```python
from build123d import *

# Parameters (mm, degrees)
SKETCH1_W               = 19.304
SKETCH1_H               = 19.304
BOSS_EXTRUDE1_DEPTH     = 203.2
CUT_EXTRUDE1_DEPTH      = 207.350575478
CUT_EXTRUDE1_DEPTH_BACK = 207.350575478


with BuildPart() as part:
    # Sketch1 → Boss-Extrude1 (new body)
    with BuildSketch(Plane(origin=(0, 0, 0), x_dir=(0, 0, -1), z_dir=(1, 0, 0))):
        with BuildLine():
            Line((0, 2.54), (0, 22.86))
            ThreePointArc((0, 22.86), (-0.743948776, 24.656051224), (-2.54, 25.4))
            Line((-2.54, 25.4), (-22.86, 25.4))
            ThreePointArc((-22.86, 25.4), (-24.656051224, 24.656051224), (-25.4, 22.86))
            Line((-25.4, 22.86), (-25.4, 2.54))
            ThreePointArc((-25.4, 2.54), (-24.656051224, 0.743948776), (-22.86, 0))
            Line((-22.86, 0), (-2.54, 0))
            ThreePointArc((-2.54, 0), (-0.743948776, 0.743948776), (0, 2.54))
        make_face()
        with Locations((-12.7, 12.7)):
            Rectangle(SKETCH1_W, SKETCH1_H, mode=Mode.SUBTRACT)
    extrude(amount=BOSS_EXTRUDE1_DEPTH)

    # Sketch2 → Cut-Extrude1 (cut, two sides: drawn at the far end of the back side and taken through both)
    with BuildSketch(Plane(origin=(0, 25.4, 0), x_dir=(1, 0, 0), z_dir=(0, 1, 0)).offset(-CUT_EXTRUDE1_DEPTH_BACK)):
        with BuildLine():
            Line((203.2, -11.1125), (174.199630657, -11.1125))
            ThreePointArc((174.199630657, -11.1125), (168.275, -12.7), (174.199630657, -14.2875))
            Line((174.199630657, -14.2875), (203.2, -14.2875))
            Line((203.2, -14.2875), (203.2, -11.1125))
        make_face()
    extrude(amount=CUT_EXTRUDE1_DEPTH + CUT_EXTRUDE1_DEPTH_BACK, mode=Mode.SUBTRACT)


solid = part.part
```
Work out the finished part from the listing and answer in its coordinate system (mm). A direction names the side the tool comes from. Give positions to 0.01 mm unless a question says otherwise; leave off trailing zeros. Loops run counter-clockwise (first coordinate to the right, second up) from the corner with the lowest first, then second, coordinate; pieces in that order, holes last. Notation, with made-up numbers: (37, 31.5) -> (72, 31.5) arc R7 ccw to (72, 37.5) -> close; hole circle Ø9 at (15, 76.25). An arc over 180 degrees is marked (long way). Write item = value, one per line. Start each with the question number.
(1) Find the intervals of material crossed by probe 1 along Z at (x, y) = (114.5, 4.5); probe 2 along X at (y, z) = (2.15, 12.7) (3 decimals), in increasing order. Write a range as from..to.
(2) The mould has two halves that part along X. Classify faces 1 (the cylindrical face through (168.277, 1.503, 12.584)), 2 (the flat face through (100, 13, 25.4)), 3 (the flat face through (203.2, 13, 24)): +X half, -X half, draft (parallel to the pull), parting line (faces both ways), or undercut.
(3) Which of the six approach directions +Z, -Z, +X, -X, +Y, -Y give full straight-line access (tool end or side, diameter ignored) to faces 4 (the flat face through (100, 13, 0)), 5 (the flat face through (100, 3.048, 13))?
(4) Find section D-D on x = 25. Give the vertices of the cut face in (y, z), and give its area (3 significant figures).
(5) Find section A-A on x = 171.45. Give the vertices of the cut face in (y, z) (3 decimals).
(6) Given pin 1 Ø2.5 at (x, y) = (185.5, 2) entering from +Z; pin 2 Ø1 at (y, z) = (16.5, 21) entering from +X; pin 3 Ø0.9 at (x, y) = (193, 1.5) entering from -Z, each flat-ended and moving along its own axis, determine where each tip first touches the part or whether it passes through.
(7) Find section B-B on z = 18.5. Give the vertices of the cut face in (x, y), and give its area (3 significant figures).
From the geometry:
q1.probe_1 = 0..3.05, 22.35..25.4
q1.probe_2 = 0..168.275
q2.face_1 = undercut
q2.face_2 = draft
q2.face_3 = +X half
q3.face_4 = -Z, +X, -X, +Y, -Y
q3.face_5 = +X, -X
q4.outline = (0, 2.54) arc R2.54 ccw to (2.54, 0) -> (22.86, 0) arc R2.54 ccw to (25.4, 2.54) -> (25.4, 22.86) arc R2.54 ccw to (22.86, 25.4) -> (2.54, 25.4) arc R2.54 ccw to (0, 22.86) -> close; hole (3.05, 3.05) -> (22.35, 3.05) -> (22.35, 22.35) -> (3.05, 22.35) -> close
q4.area = 267 mm^2
q5.outline = (0, 2.54) arc R2.54 ccw to (2.54, 0) -> (22.86, 0) arc R2.54 ccw to (25.4, 2.54) -> (25.4, 9.525) -> (22.352, 9.525) -> (22.352, 3.048) -> (3.048, 3.048) -> (3.048, 9.525) -> (0, 9.525) -> close; (0, 15.875) -> (3.048, 15.875) -> (3.048, 22.352) -> (22.352, 22.352) -> (22.352, 15.875) -> (25.4, 15.875) -> (25.4, 22.86) arc R2.54 ccw to (22.86, 25.4) -> (2.54, 25.4) arc R2.54 ccw to (0, 22.86) -> close
q6.pin_1 = 25.4
q6.pin_2 = through
q6.pin_3 = 0.07
q7.outline = (0, 0) -> (203.2, 0) -> (203.2, 3.05) -> (0, 3.05) -> close; (0, 22.35) -> (203.2, 22.35) -> (203.2, 25.4) -> (0, 25.4) -> close
q7.area = 1,240 mm^2
